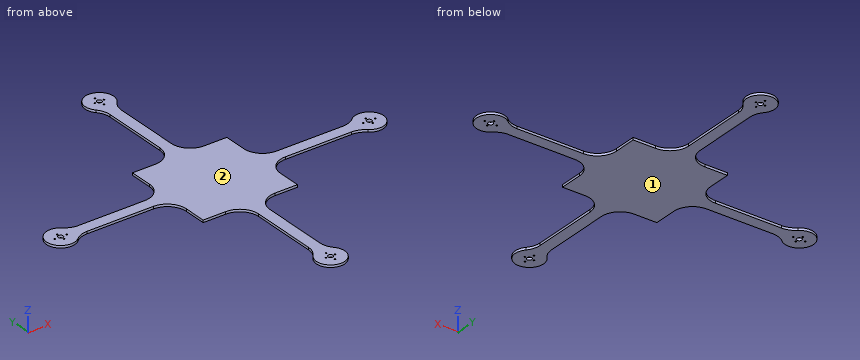
```python
from build123d import *

# Parameters (mm, degrees)
F0_R     = 1.5
F0_R_2   = 5.25
F1_DEPTH = 5


with BuildPart() as f1:
    # F0 (on Top) → F1 (new body)
    with BuildSketch(Plane.XY):
        with BuildLine():
            Line((52.176812, -100), (100, -100))
            Line((100, -100), (100, -52.176812))
            ThreePointArc((100, -52.176812), (111.715729, -23.89254), (140, -12.176812))
            Line((140, -12.176812), (280.753058, -12.176812))
            ThreePointArc((280.753058, -12.176812), (295.025184, -14.809628), (307.418515, -22.361491))
            ThreePointArc((307.418515, -22.361491), (357.417609, 0), (307.418515, 22.361491))
            ThreePointArc((307.418515, 22.361491), (295.025184, 14.809628), (280.753058, 12.176812))
            Line((280.753058, 12.176812), (140, 12.176812))
            ThreePointArc((140, 12.176812), (111.715729, 23.89254), (100, 52.176812))
            Line((100, 52.176812), (100, 100))
            Line((100, 100), (52.176812, 100))
            ThreePointArc((52.176812, 100), (23.89254, 111.715729), (12.176812, 140))
            Line((12.176812, 140), (12.176812, 280.753058))
            ThreePointArc((12.176812, 280.753058), (14.809628, 295.025184), (22.361491, 307.418515))
            ThreePointArc((22.361491, 307.418515), (0, 357.417609), (-22.361491, 307.418515))
            ThreePointArc((-22.361491, 307.418515), (-14.809628, 295.025184), (-12.176812, 280.753058))
            Line((-12.176812, 280.753058), (-12.176812, 140))
            ThreePointArc((-12.176812, 140), (-23.89254, 111.715729), (-52.176812, 100))
            Line((-52.176812, 100), (-100, 100))
            Line((-100, 100), (-100, 52.176812))
            ThreePointArc((-100, 52.176812), (-111.715729, 23.89254), (-140, 12.176812))
            Line((-140, 12.176812), (-280.753058, 12.176812))
            ThreePointArc((-280.753058, 12.176812), (-295.025184, 14.809628), (-307.418515, 22.361491))
            ThreePointArc((-307.418515, 22.361491), (-357.417609, 0), (-307.418515, -22.361491))
            ThreePointArc((-307.418515, -22.361491), (-295.025184, -14.809628), (-280.753058, -12.176812))
            Line((-280.753058, -12.176812), (-140, -12.176812))
            ThreePointArc((-140, -12.176812), (-111.715729, -23.89254), (-100, -52.176812))
            Line((-100, -52.176812), (-100, -100))
            Line((-100, -100), (-52.176812, -100))
            ThreePointArc((-52.176812, -100), (-23.89254, -111.715729), (-12.176812, -140))
            Line((-12.176812, -140), (-12.176812, -280.753058))
            ThreePointArc((-12.176812, -280.753058), (-14.809628, -295.025184), (-22.361491, -307.418515))
            ThreePointArc((-22.361491, -307.418515), (0, -357.417609), (22.361491, -307.418515))
            ThreePointArc((22.361491, -307.418515), (14.809628, -295.025184), (12.176812, -280.753058))
            Line((12.176812, -280.753058), (12.176812, -140))
            ThreePointArc((12.176812, -140), (23.89254, -111.715729), (52.176812, -100))
        make_face()
        with Locations((-0.023046, -340.050671)):
            Circle(F0_R, mode=Mode.SUBTRACT)
        with Locations((-9.522677, -327.350178)):
            Circle(F0_R, mode=Mode.SUBTRACT)
        with Locations((-0.023046, -314.650178)):
            Circle(F0_R, mode=Mode.SUBTRACT)
        with Locations((-340.050671, -0.023046)):
            Circle(F0_R, mode=Mode.SUBTRACT)
        with Locations((-327.350178, -9.522677)):
            Circle(F0_R, mode=Mode.SUBTRACT)
        with Locations((-314.650178, -0.023046)):
            Circle(F0_R, mode=Mode.SUBTRACT)
        with Locations((0, -327.417609)):
            Circle(F0_R_2, mode=Mode.SUBTRACT)
        with Locations((9.476954, -327.350178)):
            Circle(F0_R, mode=Mode.SUBTRACT)
        with Locations((327.350178, -9.476954)):
            Circle(F0_R, mode=Mode.SUBTRACT)
        with Locations((-327.417609, 0)):
            Circle(F0_R_2, mode=Mode.SUBTRACT)
        with Locations((-327.350178, 9.476954)):
            Circle(F0_R, mode=Mode.SUBTRACT)
        with Locations((-9.476954, 327.350178)):
            Circle(F0_R, mode=Mode.SUBTRACT)
        with Locations((314.650178, 0.023046)):
            Circle(F0_R, mode=Mode.SUBTRACT)
        with Locations((327.417609, 0)):
            Circle(F0_R_2, mode=Mode.SUBTRACT)
        with Locations((327.350178, 9.522677)):
            Circle(F0_R, mode=Mode.SUBTRACT)
        with Locations((340.050671, 0.023046)):
            Circle(F0_R, mode=Mode.SUBTRACT)
        with Locations((0.023046, 314.650178)):
            Circle(F0_R, mode=Mode.SUBTRACT)
        with Locations((0, 327.417609)):
            Circle(F0_R_2, mode=Mode.SUBTRACT)
        with Locations((9.522677, 327.350178)):
            Circle(F0_R, mode=Mode.SUBTRACT)
        with Locations((0.023046, 340.050671)):
            Circle(F0_R, mode=Mode.SUBTRACT)
    extrude(amount=F1_DEPTH)


solid = f1.part
```
Input: part model. Units: mm. Frame: model coordinates. Face numbers are marked on the shaded views. Coordinates: 2 decimals unless noted, no trailing zeros. Write each loop counter-clockwise with the first axis right and the second up, starting at its lowest first coordinate (ties: lowest second). Pieces come first, ordered by that corner, then holes.
1) Mould query, pull axis Z, two halves, no side actions, for the marked faces 1 and 2. Classes: pulls with the +Z half, pulls with the -Z half, needs draft (parallel to the pull), parting line crosses it, or undercut.
2) Section A-A on y = -75. Output: boundary loops of the cut face in (x, z).
3) Section C-C on x = 151.5. Output: boundary loops of the cut face in (y, z), and give its area (3 significant figures).
4) Material intervals for line 1 along X through (y, z) = (76, 2.5); line 2 along X through (y, z) = (225, 1.1), sorted ascending.
5) Section B-B on z = 2.5. State how many separate pieces and enclosed holes the cut face has, and give its area (3 significant figures).
6) Pin query (flat end, axial travel): pin 1 Ø9.5 at (x, y) = (0, -327.42) entering from -Z; pin 2 Ø1.5 at (x, z) = (-193, 4) entering from -Y; pin 3 Ø2.5 at (y, z) = (-85.5, 2.5) entering from +X; pin 4 Ø1.5 at (x, z) = (-198, 2.5) entering from +Y. Return the tip coordinate at first contact, or that it passes through.
Check result:
1. face 1: pulls with the -Z half
1. face 2: pulls with the +Z half
2. outline: (-100, 0) - (100, 0) - (100, 5) - (-100, 5) - close
3. outline: (-12.18, 0) - (12.18, 0) - (12.18, 5) - (-12.18, 5) - close
3. area: 122 mm2
4. line 1: x = -100 to 100
4. line 2: x = -12.18 to 12.18
5. separate pieces: 1
5. enclosed holes: 20
5. area: 73,200 mm2
6. pin 1: passes through
6. pin 2: stops at y = -12.18
6. pin 3: stops at x = 100
6. pin 4: stops at y = 12.18
